Autodesk Inventor part; units mm, degrees
ref_plane "YZ Plane" through (0, 0, 0) normal (1, 0, 0) x (0, 1, 0)
ref_plane "XZ Plane" through (0, 0, 0) normal (0, 1, 0) x (-1, 0, 0)
ref_plane "XY Plane" through (0, 0, 0) normal (0, 0, 1) x (1, 0, 0)
sketch "Sketch1" plane through (0, 0, 0) normal (1, 0, 0) x (0, 1, 0)
  line L0 (10.279, 12) -> (9.5154, 12)
  line L1 (9.5154, 12) -> (9.5154, 10.3)
  line L2 (9.5154, 10.3) -> (10.5154, 10.3)
  line L3 (10.5154, 10.3) -> (10.5154, 11)
  line L4 (10.5154, 11) -> (12.1654, 11)
  line L5 (13.1654, 12) -> (10.279, 12)
  line L6 (13.1654, 12) -> (13.1654, 1)
  line L7 (12.1654, 1) -> (12.1654, 11)
  line L8 (12.1654, 1) -> (1, 1)
  line L9 (0, 1.2006) -> (0, 0)
  line L10 (0, 0) -> (13.1654, 0)
  line L11 (13.1654, 0) -> (13.1654, 1)
  line L12 (0, 1.2006) -> (0, 2.9)
  line L13 (0, 2.9) -> (1, 2.9)
  line L14 (1, 2.9) -> (1, 1)
  dimension "d0" = 0.7
  dimension "d1" = 1.65
  dimension "d2" = 10
  dimension "d3" = 11.1654
  dimension "d4" = 1
  dimension "d5" = 1
  dimension "d6" = 1
  dimension "d7" = 1
  dimension "d8" = 1
  dimension "d9" = 1.9
extrude "Extrusion1" add sketch "Sketch1" along normal blind 5
fillet "Fillet1" radius 0.5 6 edges at (2.5, 9.5154, 10.3) (2.5, 9.5154, 12) (2.5, 13.1654, 12) (2.5, 13.1654, 0) (2.5, 0, 0) (2.5, 0, 2.9)
sketch "Sketch2" plane through (5, 0, 0) normal (1, 0, 0) x (0, 0, -1)
  line L0 (-0.5, 13.1654) -> (-11.5, 13.1654)
  line L1 (-11.5, 13.1654) -> (-10.5, 13.1654)
  line L2 (-10.5, 13.1654) -> (-10.5, 17.1654)
  line L3 (-10.5, 17.1654) -> (-11.5, 17.1654)
  line L4 (-11.5, 17.1654) -> (-11.5, 13.1654)
  line L5 (-0.5, 18.1654) -> (-1.5, 18.1654)
  line L6 (-1.5, 18.1654) -> (-1.5, 13.1654)
  line L7 (-1.5, 13.1654) -> (-0.5, 13.1654)
  line L8 (-0.5, 13.1654) -> (-0.5, 18.1654)
  point P0 (0, 0)
  dimension "d13" = 10
  dimension "d14" = 1
  dimension "d15" = 1
  dimension "d16" = 5
  dimension "d17" = 4
extrude "Extrusion2" add sketch "Sketch2" against normal blind 5
fillet "Fillet2" radius 0.5 8 edges at (2.5, 13.1654, 10.5) (2.5, 13.1654, 11.5) (2.5, 17.1654, 11.5) (2.5, 17.1654, 10.5) (2.5, 13.1654, 1.5) (2.5, 18.1654, 1.5) (2.5, 18.1654, 0.5) (2.5, 13.1654, 0.5)
properties part number "monitor-clip"
CAD build for the part. Positions are in the model's coordinates, mm. A direction names the side the tool comes from. Give positions to 0.01 mm unless a question says otherwise; leave off trailing zeros. Loops run counter-clockwise (first coordinate to the right, second up) from the corner with the lowest first, then second, coordinate; pieces in that order, holes last. Notation, with made-up numbers: M 62,15 L 110,15 A24 ccw 110,48 Z; hole C 81.25,88.5 d5. An arc over 180 degrees is marked long. Write each question's results on one line, items separated by ' | '.
Q1. Band-saw the part on B-B on z = 1.25. Write the cut outline in (x, y).
Geometry check:
outline: M 0,0 L 5,0 L 5,1 L 0,1 Z; M 0,12.17 L 5,12.17 L 5,18.1 L 0,18.1 Z
Q2. Band-saw the part on A-A on y = 15.75. Write the cut outline in (x, z), and give its area (3 significant figures).
Geometry check:
outline: M 0,0.5 L 5,0.5 L 5,1.5 L 0,1.5 Z; M 0,10.5 L 5,10.5 L 5,11.5 L 0,11.5 Z | area: 10.0 mm²
Q3. Mould opens along Y. For faces 1 (the face through (2, 12.165, 6)), 2 (the face through (2, 0, 1)), 3 (the face through (3, 15, 10.5)) say: pulls with the +Y half, pulls with the -Y half, needs draft (parallel to the pull), parting line crosses it, or undercut.
Geometry check:
face 1: undercut | face 2: pulls with the -Y half | face 3: needs draft
Q4. Which spindle directions (+Z, -Z, +X, -X, +Y, -Y) get a long thin tool onto all of the face, cutting with end or side? Do faces 4 (the face through (2, 1, 2)), 5 (the face through (3, 16, 1.5)), 6 (the face through (2, 11, 11)). Say none if no direction does.
Geometry check:
face 4: +Z, +X, -X | face 5: +X, -X, +Y | face 6: +X, -X
Q5. Probe probe 1 along Z at (x, y) = (2.9, 12); probe 2 along Y at (x, z) = (3.7, 2); probe 3 along Z at (x, y) = (3.9, 4.25). List the from-to ranges inside material, lowest first.
Geometry check:
probe 1: z = 0 to 1, 11 to 12 | probe 2: y = 0 to 1, 12.17 to 13.17 | probe 3: z = 0 to 1
Q6. Band-saw the part on D-D on y = 2.75. Write the cut outline in (x, z).
Geometry check:
outline: M 0,0 L 5,0 L 5,1 L 0,1 Z
Q7. Flat gauge pins, fed straight in: P1, Ø0.6, axis at x = 1.5, z = 11, coming from the -Y side; P2, Ø1, axis at x = 3, z = 9.5, coming from the -Y side; P3, Ø1, axis at x = 1.5, y = 4, coming from the -Z side; P4, Ø3, axis at x = 2, z = 10.5, coming from the +Y side. Where does each tip first touch, or does it go through?
Geometry check:
P1: stops at y = 9.52 | P2: stops at y = 12.17 | P3: stops at z = 0 | P4: stops at y = 17.17
